The model under review builds one solid part; all positions refer to its coordinate system, in mm. Give positions to 0.01 mm unless a question says otherwise; leave off trailing zeros. Loops run counter-clockwise (first coordinate to the right, second up) from the corner with the lowest first, then second, coordinate; pieces in that order, holes last. Notation, with made-up numbers: M 32,39 L 43,39 A12 cw 43,48 Z; hole C 80,60.5 d2. An arc over 180 degrees is marked long. Return JSON: item names as keys, results as strings. Group by question number.
```python
from build123d import *

# Parameters (mm, degrees)
F1_DEPTH      = 150
F1_DEPTH_BACK = 125
F3_DEPTH      = 2000


with BuildPart() as f1:
    # F0 (on Right) → F1 (new body, two sides)
    with BuildSketch(Plane.YZ) as f1_sk:
        Polygon((-150, 20), (-150, 0), (350, 0), (350, 60), (265.2117013931, 69.0981149673), (240.4940045903, 100), (90.4940045903, 100), (0, 51.8834842505), align=None)
    extrude(amount=F1_DEPTH)
    extrude(f1_sk.sketch, amount=-F1_DEPTH_BACK)

    # F2 (on face) → F3 (intersect)
    with BuildSketch(Plane(origin=(0, 350, 0), x_dir=(-1, 0, 0), z_dir=(0, 1, 0))):
        Polygon((122.7646524241, 59.4295346152), (80, 100), (-105, 100), (-127.2353475759, 59.4295346152), (-150, 20), (-150, 0), (125, 0), (125, 20), align=None)
    extrude(amount=-F3_DEPTH, mode=Mode.INTERSECT)


solid = f1.part
```
(1) Add section A-A (x = -66.5). Write out the cut boundary in (y, z).
(2) Add section D-D (y = -81). Write out the cut boundary in (x, z), and give its area (3 significant figures).
(3) Add section B-B (y = 172). Write out the cut boundary in (x, z), and give its area (3 significant figures).
(4) For pin 1 (2 mm diameter, centred on x = 15.5, y = 32.5, fed in from +Z); pin 2 (6 mm diameter, centred on x = -46, y = 279, fed in from +Z), all flat-tipped, find the tip position at first contact; note any pin that passes through.
(5) For probe 1 along X at (y, z) = (5, 22); probe 2 along Z at (x, y) = (73.5, -15); probe 3 along X at (y, z) = (208, 64), list the stretches that pass through material, from the lowest coordinate up.
(6) Add section C-C (z = 94). Write out the cut boundary in (x, y), and give its area (3 significant figures).
Verdict:
{
 "1": {"outline": "M -150,0 L 350,0 L 350,60 L 265.21,69.1 L 240.49,100 L 90.49,100 L 0,51.88 L -150,20 Z"},
 "2": {"outline": "M -125,0 L 150,0 L 150,20 L 141.53,34.67 L -124.17,34.67 L -125,20 Z", "area": "9,470 mm²"},
 "3": {"outline": "M -125,0 L 150,0 L 150,20 L 127.24,59.43 L 105,100 L -80,100 L -122.76,59.43 L -125,20 Z", "area": "24,700 mm²"},
 "4": {"pin 1": "stops at z = 69.7", "pin 2": "stops at z = 67.94"},
 "5": {"probe 1": "x = -124.89 to 148.85", "probe 2": "z = 0 to 48.7", "probe 3": "x = -117.95 to 124.73"},
 "6": {"outline": "M -86.32,79.21 L 108.29,79.21 L 108.29,245.29 L -86.32,245.29 Z", "area": "32,300 mm²"}
}
